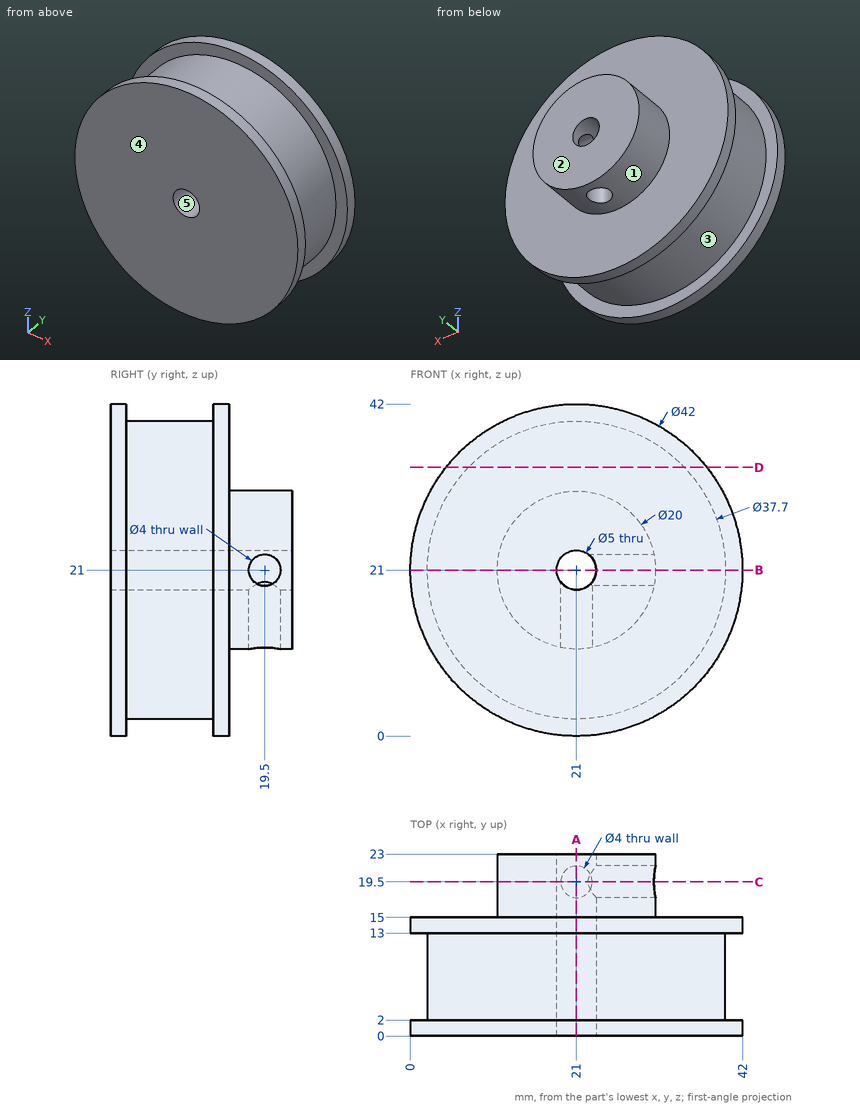
Input: dimensioned drawing with shaded views. Units: mm. Origin: part minimum x, y, z. A direction names the side the tool comes from. Round coordinates to 2 decimals unless told otherwise and drop trailing zeros. Order: outer loops, then holes, each group sorted by start corner. A loop starts at its lowest first (then second) coordinate and runs counter-clockwise, first axis right, second up.
Q1. Material intervals for probe 1 along X at (y, z) = (17, 21); probe 2 along Y at (x, z) = (21, 13.5); probe 3 along Z at (x, y) = (21, 11.75), sorted ascending.
Result sheet:
probe 1: x = 11 to 18.5, 23.5 to 31
probe 2: y = 0 to 17.5, 21.5 to 23
probe 3: z = 2.15 to 18.5, 23.5 to 39.85
Q2. Section A-A, the plane x = 21. Output: boundary loops of the cut face in (y, z).
Result sheet:
outline: (0, 0) - (2, 0) - (2, 2.15) - (13, 2.15) - (13, 0) - (15, 0) - (15, 11) - (17.5, 11) - (17.5, 18.5) - (0, 18.5) - close; (0, 23.5) - (23, 23.5) - (23, 31) - (15, 31) - (15, 42) - (13, 42) - (13, 39.85) - (2, 39.85) - (2, 42) - (0, 42) - close; (21.5, 11) - (23, 11) - (23, 18.5) - (21.5, 18.5) - close
Q3. Section C-C, the plane y = 19.5. Output: boundary loops of the cut face in (x, z), and give its area (3 significant figures).
Result sheet:
outline: (19, 11.2) - (19, 19.5) arc R2.5 cw to (22.5, 23) - (30.8, 23) arc R10 ccw (long way) to start; (23, 11.2) arc R10 ccw to (30.8, 19) - (23, 19) - close
area: 233 mm2
Q4. Mould query, pull axis X, two halves, no side actions, for the marked faces 3, 4 and 5. Classes: released by +X, released by -X, zero draft, split by the parting line, or undercut.
Result sheet:
face 3: split by the parting line
face 4: zero draft
face 5: undercut
Q5. Section D-D, the plane z = 34. Output: boundary loops of the cut face in (x, y).
Result sheet:
outline: (4.51, 0) - (37.49, 0) - (37.49, 2) - (34.65, 2) - (34.65, 13) - (37.49, 13) - (37.49, 15) - (4.51, 15) - (4.51, 13) - (7.35, 13) - (7.35, 2) - (4.51, 2) - close
Q6. Access query for the marked faces 1 and 2. Directions: +Z, -Z, +X, -X, +Y, -Y. A direction counts if a zero-diameter tool reaches every point of the face in a straight line with its end or side. Return the directions, or none.
Result sheet:
face 1: +Y
face 2: +Z, -Z, +X, -X, +Y
Q7. Pin query (flat end, axial travel): pin 1 (6.5 mm diameter, centred on x = 21, y = 19.5, fed in from +Z); pin 2 (12 mm diameter, centred on y = 7.5, z = 31.5, fed in from +X); pin 3 (5 mm diameter, centred on y = 19.5, z = 21, fed in from +X). Return the tip coordinate at first contact, or that it passes through.
Result sheet:
pin 1: stops at z = 31
pin 2: stops at x = 40.37
pin 3: stops at x = 31
Q8. Section B-B, the plane z = 21. Output: boundary loops of the cut face in (x, y), and give its area (3 significant figures).
Result sheet:
outline: (0, 0) - (18.5, 0) - (18.5, 23) - (11, 23) - (11, 15) - (0, 15) - (0, 13) - (2.15, 13) - (2.15, 2) - (0, 2) - close; (23.5, 0) - (42, 0) - (42, 2) - (39.85, 2) - (39.85, 13) - (42, 13) - (42, 15) - (31, 15) - (31, 17.5) - (23.5, 17.5) - close; (23.5, 21.5) - (31, 21.5) - (31, 23) - (23.5, 23) - close
area: 598 mm2
